The model under review builds one solid part; all positions refer to its coordinate system, in mm. Give positions to 0.01 mm unless a question says otherwise; leave off trailing zeros. Write each loop counter-clockwise with the first axis right and the second up, starting at its lowest first coordinate (ties: lowest second). Pieces come first, ordered by that corner, then holes.
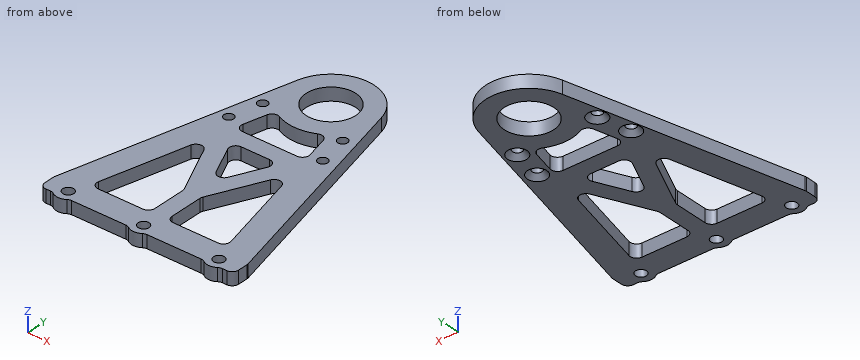
from build123d import *

# Parameters (mm, degrees)
SKETCH_1_R                   = 20
SKETCH_1_R_2                 = 11.5
EXTRUDE_1_DEPTH              = 6
SKETCH_5_W                   = 90
SKETCH_5_H                   = 8
EXTRUDE_2_DEPTH              = 6
SKETCH_6_R                   = 2.1
CUT_EXTRUDE_1_DEPTH          = 129.300428682
HOLE_WIZARD_M4_1_D           = 4.5
HOLE_WIZARD_M4_1_DEPTH       = 11.4
HOLE_WIZARD_M4_1_CSINK_D     = 8.96
HOLE_WIZARD_M4_1_CSINK_ANGLE = 90
HOLE_WIZARD_M4_1_TIP         = 1.351936393
SKETCH_10_R                  = 2.55
CUT_EXTRUDE_2_DEPTH          = 129.300428682
EXTRUDE_4_DEPTH              = 6
CUT_EXTRUDE_3_DEPTH          = 129.300428682
FILLET_1_R                   = 3


with BuildPart() as part:
    # 草图1 → 凸台-拉伸1 (new body)
    # profile 1 of 3: a face of its own
    with BuildSketch(Plane.XY):
        with Locations((0, 100)):
            Circle(SKETCH_1_R)
        with Locations((0, 100)):
            Circle(SKETCH_1_R_2, mode=Mode.SUBTRACT)
    # profile 2 of 3: a face of its own
    with BuildSketch(Plane.XY):
        with BuildLine():
            Line((-19.429404285, 104.743231928), (-45, 0))
            Line((-45, 0), (45, 0))
            Line((45, 0), (19.429404285, 104.743231928))
            ThreePointArc((19.429404285, 104.743231928), (19.856838692, 102.388714539), (20, 100))
            ThreePointArc((20, 100), (-2.388714539, 80.143161308), (-19.429404285, 104.743231928))
        make_face()
    # profile 3 of 3: a face of its own
    with BuildSketch(Plane.XY):
        with BuildLine():
            Line((-19.429404285, 104.743231928), (-45, 0))
            Line((-45, 0), (45, 0))
            Line((45, 0), (19.429404285, 104.743231928))
            ThreePointArc((19.429404285, 104.743231928), (19.856838692, 102.388714539), (20, 100))
            ThreePointArc((20, 100), (-2.388714539, 80.143161308), (-19.429404285, 104.743231928))
        make_face()
    extrude(amount=EXTRUDE_1_DEPTH)

    # 草图5 → 凸台-拉伸2 (add)
    with BuildSketch(Plane.XY.offset(6)):
        with Locations((0, -4)):
            Rectangle(SKETCH_5_W, SKETCH_5_H)
    extrude(amount=-EXTRUDE_2_DEPTH)

    # 草图6 → 切除-拉伸1 (cut, through all)
    with BuildSketch(Plane.XY.offset(6)):
        with Locations((-22.667866245, 70.382755655)):
            Circle(SKETCH_6_R)
        with Locations((21.643312936, 69.625992562)):
            Circle(SKETCH_6_R)
        with Locations((18.58555253, 84.311022398)):
            Circle(SKETCH_6_R)
        with Locations((-19.110442299, 84.954808869)):
            Circle(SKETCH_6_R)
    extrude(amount=-CUT_EXTRUDE_1_DEPTH, mode=Mode.SUBTRACT)

    # M4 六角凹锥坑螺钉的锥形沉头孔1
    with Locations(Plane(origin=(0, 0, 0), x_dir=(-1, 0, 0), z_dir=(0, 0, -1))):
        with Locations((22.667866245, 70.382755655), (19.110442299, 84.954808869), (-18.58555253, 84.311022398), (-21.643312936, 69.625992562)):
            CounterSinkHole(HOLE_WIZARD_M4_1_D / 2, HOLE_WIZARD_M4_1_CSINK_D / 2, depth=HOLE_WIZARD_M4_1_DEPTH, counter_sink_angle=HOLE_WIZARD_M4_1_CSINK_ANGLE)
            with Locations((0, 0, -(HOLE_WIZARD_M4_1_DEPTH + HOLE_WIZARD_M4_1_TIP / 2))):  # 118° drill point
                Cone(0, HOLE_WIZARD_M4_1_D / 2, HOLE_WIZARD_M4_1_TIP, mode=Mode.SUBTRACT)

    # 草图10 → 切除-拉伸2 (cut, through all)
    with BuildSketch(Plane(origin=(0, 0, 0), x_dir=(-1, 0, 0), z_dir=(0, 0, -1))):
        with Locations((-35, -4)):
            Circle(SKETCH_10_R)
        with Locations((0, -4)):
            Circle(SKETCH_10_R)
        with Locations((35, -4)):
            Circle(SKETCH_10_R)
    extrude(amount=-CUT_EXTRUDE_2_DEPTH, mode=Mode.SUBTRACT)

    # 草图11 → 凸台-拉伸4 (add)
    with BuildSketch(Plane(origin=(0, 0, 0), x_dir=(-1, 0, 0), z_dir=(0, 0, -1))):
        with BuildLine():
            Line((-31.152598279, -8), (-38.847401721, -8))
            ThreePointArc((-38.847401721, -8), (-35, -9.55), (-31.152598279, -8))
        make_face()
        with BuildLine():
            Line((3.847401721, -8), (-3.847401721, -8))
            ThreePointArc((-3.847401721, -8), (0, -9.55), (3.847401721, -8))
        make_face()
        with BuildLine():
            ThreePointArc((31.152598279, -8), (35, -9.55), (38.847401721, -8))
            Line((38.847401721, -8), (31.152598279, -8))
        make_face()
    extrude(amount=-EXTRUDE_4_DEPTH)

    # 草图9 → 切除-拉伸3 (cut, through all)
    with BuildSketch(Plane(origin=(0, 0, 0), x_dir=(-1, 0, 0), z_dir=(0, 0, -1))):
        with BuildLine():
            ThreePointArc((12.119005584, 84.089949602), (0, 80), (-12.119005584, 84.089949602))
            Line((-12.119005584, 84.089949602), (-16.535241166, 66))
            Line((-16.535241166, 66), (16.535241166, 66))
            Line((16.535241166, 66), (12.119005584, 84.089949602))
        make_face()
        Polygon((11.264099529, 58), (-11.264099529, 58), (0, 33.55721992), align=None)
        Polygon((-4, 23.122667902), (-19.036946629, 55.752420381), (-31.671082453, 4), (-4, 4), align=None)
        Polygon((31.671082453, 4), (19.036946629, 55.752420381), (4, 23.122667902), (4, 4), align=None)
    extrude(amount=-CUT_EXTRUDE_3_DEPTH, mode=Mode.SUBTRACT)

    # 圆角1
    fillet_1_edges = [part.edges().sort_by_distance(p)[0] for p in [
        (45, 0, 3),
        (-45, 0, 3),
        (31.152598279, -8, 3),
        (38.847401721, -8, 3),
        (-3.847401721, -8, 3),
        (3.847401721, -8, 3),
        (-38.847401721, -8, 3),
        (-31.152598279, -8, 3),
        (12.119005584, 84.089949602, 3),
        (-12.119005584, 84.089949602, 3),
        (-16.535241166, 66, 3),
        (16.535241166, 66, 3),
        (-4, 23.122667902, 3),
        (-19.036946629, 55.752420381, 3),
        (-31.671082453, 4, 3),
        (-4, 4, 3),
        (11.264099529, 58, 3),
        (-11.264099529, 58, 3),
        (0, 33.55721992, 3),
        (4, 23.122667902, 3),
        (4, 4, 3),
        (31.671082453, 4, 3),
        (19.036946629, 55.752420381, 3),
        (-45, -8, 3),
        (45, -8, 3),
    ]]
    fillet(fillet_1_edges, radius=FILLET_1_R)


solid = part.part
1) Consider section D-D, the plane z = 1. State how many separate pieces and enclosed holes the cut face has, then the cut area to 3 significant figures.
2) To check wall thickness, follow probe 1 along Y at (x, z) = (0, 3.7); probe 2 along X at (y, z) = (31, 2.5); probe 3 along X at (y, z) = (25, 1.5). State the ranges of each line that lie inside material, in increasing order.
3) Consider section A-A, the plane x = 0. Give the boundary of the cut face in (y, z), then the cut area to 3 significant figures.
4) Consider section B-B, the plane y = 100. Give the boundary of the cut face in (x, z), then the cut area to 3 significant figures.
5) Insertion check: pin 1 (1.8 mm diameter, centred on x = 15.5, z = 2, fed in from -Y); pin 2 (6 mm diameter, centred on x = 18.59, y = 84.31, fed in from -Z); pin 3 (1.5 mm diameter, centred on x = 9, y = 102.5, fed in from +Z); pin 4 (8 mm diameter, centred on x = -35, y = -4, fed in from -Z). Each pin has a flat end and moves straight along its axis. Give the tip position at first contact, or say it passes through.
6) Consider section C-C, the plane x = -35. Give the boundary of the cut face in (y, z), then the cut area to 3 significant figures.
Answer block:
1. separate pieces: 1
1. enclosed holes: 12
1. area: 4,930 mm2
2. probe 1: y = -9.55 to -6.55, -1.45 to 37.73, 58 to 66, 80 to 88.5, 111.5 to 120
2. probe 2: x = -37.43 to -25.08, -7.63 to 7.63, 25.08 to 37.43
2. probe 3: x = -38.9 to -26.54, -4.87 to 4.87, 26.54 to 38.9
3. outline: (-9.55, 0) - (-6.55, 0) - (-6.55, 6) - (-9.55, 6) - close; (-1.45, 0) - (37.73, 0) - (37.73, 6) - (-1.45, 6) - close; (58, 0) - (66, 0) - (66, 6) - (58, 6) - close; (80, 0) - (88.5, 0) - (88.5, 6) - (80, 6) - close; (111.5, 0) - (120, 0) - (120, 6) - (111.5, 6) - close
3. area: 403 mm2
4. outline: (-20.59, 0) - (-11.5, 0) - (-11.5, 6) - (-20.59, 6) - close; (11.5, 0) - (20.59, 0) - (20.59, 6) - (11.5, 6) - close
4. area: 109 mm2
5. pin 1: stops at y = -8
5. pin 2: stops at z = 1.48
5. pin 3: passes through
5. pin 4: stops at z = 0
6. outline: (-9.55, 0) - (-6.55, 0) - (-6.55, 6) - (-9.55, 6) - close; (-1.45, 0) - (40.96, 0) - (40.96, 6) - (-1.45, 6) - close
6. area: 272 mm2
